The listing builds one solid part. Answer for the finished solid, in the listing's coordinates (mm). A direction names the side the tool comes from. Round coordinates to 2 decimals unless told otherwise and drop trailing zeros. Write each loop counter-clockwise with the first axis right and the second up, starting at its lowest first coordinate (ties: lowest second). Pieces come first, ordered by that corner, then holes. Notation, with made-up numbers: M 30,12 L 89,12 A12 cw 89,24 Z; hole C -7,-21.5 d6. An arc over 180 degrees is marked long. One line per item, written item: value. Start each with the question number.
(1) Section C-C (y = 1485.5) is taken. Determine the outline of the cut face in (x, z), plus the area to 3 significant figures.
(2) Section D-D (z = -74) is taken. Determine the outline of the cut face in (x, y).
(3) Given P1, Ø6, axis at x = -84.5, z = -64.5, coming from the -Y side; P2, Ø15, axis at x = -114.5, z = 61.5, coming from the +Y side; P3, Ø1.5, axis at y = 892, z = -127, coming from the -X side; P4, Ø3, axis at y = 910, z = 92.5, coming from the +X side, each flat-ended and moving along its own axis, determine where each tip first touches the part or whether it passes through.
(4) For faces 1 (the flat face through (-114, 104.96, 4)), 2 (the flat face through (88.9, 1035, -53)), 3 (the flat face through (-2, 1288, -254)), determine the directions among +Z, -Z, +X, -X, +Y, -Y from which every point of the face is accessible in a straight line to the end or side of a thin tool.
(5) Section A-A (x = -62) is taken. Determine the outline of the cut face in (y, z).
(6) Consider probe 1 along X at (y, z) = (1894.5, -182); probe 2 along Y at (x, z) = (128, -197.5); probe 3 along Z at (x, y) = (66.5, 1653). Determine where each line is inside the solid, lowest interval first.
(7) Section B-B (z = -178) is taken. Determine the outline of the cut face in (x, y), plus the area to 3 significant figures.
```python
from build123d import *

# Parameters (mm, degrees)
BOSS_EXTRUDE1_DEPTH     = 254
CUT_EXTRUDE1_DEPTH      = 140.7
CUT_EXTRUDE1_DEPTH_BACK = 140.7


with BuildPart() as part:
    # Sketch1 → Boss-Extrude1 (new body, symmetric)
    with BuildSketch(Plane.XY):
        Polygon((88.9, 2540), (-88.9, 2540), (-88.9, 104.96042), (-139.7, 104.96042), (-139.7, 0), (139.7, 0), (139.7, 104.96042), (88.9, 104.96042), align=None)
    extrude(amount=BOSS_EXTRUDE1_DEPTH, both=True)

    # Sketch2 → Cut-Extrude1 (cut, two sides)
    with BuildSketch(Plane(origin=(0, 0, 0), x_dir=(0, 0, -1), z_dir=(1, 0, 0))) as cut_extrude1_sk:
        Polygon((-254, 104.96042), (101.6, 2540), (-254, 2540), align=None)
    extrude(amount=CUT_EXTRUDE1_DEPTH, mode=Mode.SUBTRACT)
    extrude(cut_extrude1_sk.sketch, amount=-CUT_EXTRUDE1_DEPTH_BACK, mode=Mode.SUBTRACT)


solid = part.part
```
Recorded:
1. outline: M -88.9,-254 L 88.9,-254 L 88.9,52.39 L -88.9,52.39 Z
1. area: 54,500 mm2
2. outline: M -139.7,0 L 139.7,0 L 139.7,104.96 L 88.9,104.96 L 88.9,2351 L -88.9,2351 L -88.9,104.96 L -139.7,104.96 Z
3. P1: stops at y = 0
3. P2: stops at y = 104.96
3. P3: stops at x = -88.9
3. P4: stops at x = 88.9
4. face 1: +Z, -Z, -X, +Y
4. face 2: +Z, -Z, +X, +Y
4. face 3: -Z, +X, -X, +Y, -Y
5. outline: M 0,-254 L 2540,-254 L 2540,-101.6 L 104.96,254 L 0,254 Z
6. probe 1: x = -88.9 to 88.9
6. probe 2: y = 0 to 104.96
6. probe 3: z = -254 to 27.93
7. outline: M -139.7,0 L 139.7,0 L 139.7,104.96 L 88.9,104.96 L 88.9,2540 L -88.9,2540 L -88.9,104.96 L -139.7,104.96 Z
7. area: 462,000 mm2
